CAD build for the part. Positions are in the model's coordinates, mm. Face numbers are marked on the shaded views. A direction names the side the tool comes from. Coordinates: 2 decimals unless noted, no trailing zeros. Write each loop counter-clockwise with the first axis right and the second up, starting at its lowest first coordinate (ties: lowest second). Pieces come first, ordered by that corner, then holes.
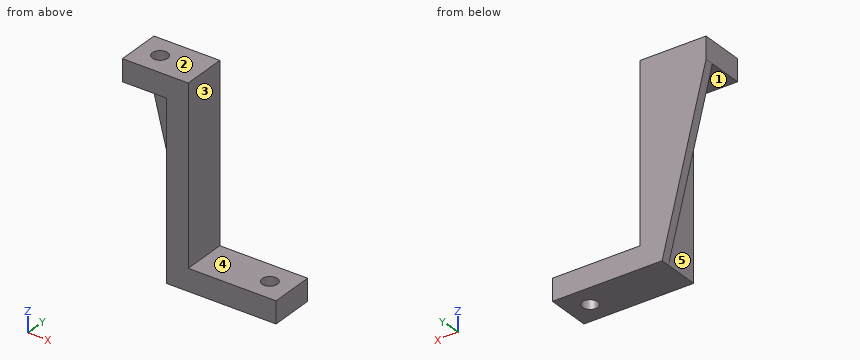
```python
from build123d import *

# Parameters (mm, degrees)
F1_DEPTH = 10
F2_DEPTH = 2
F3_R     = 1.75
F4_DEPTH = 5
F5_R     = 1.75
F6_DEPTH = 5


with BuildPart() as f1:
    # F0 (on Front) → F1 (new body)
    with BuildSketch(Plane.XZ):
        Polygon((0, 40), (-15, 40), (-15, 35), (-5, 35), (-5, -5), (20, -5), (20, 0), (0, 0), align=None)
    extrude(amount=F1_DEPTH)

    # F0 (on Front) → F2 (join)
    with BuildSketch(Plane.XZ):
        Polygon((0, 40), (-15, 40), (-15, 35), (-5, 35), (-5, -5), (20, -5), (20, 0), (0, 0), align=None)
        Polygon((-5, 35), (-15, 35), (-5, -5), align=None)
    extrude(amount=F2_DEPTH)

    # F3 (on face) → F4 (cut)
    with BuildSketch(Plane.XY.offset(40)):
        with Locations((-10, -5)):
            Circle(F3_R)
    extrude(amount=-F4_DEPTH, mode=Mode.SUBTRACT)

    # F5 (on face) → F6 (cut)
    with BuildSketch(Plane.XY):
        with Locations((15, -5)):
            Circle(F5_R)
    extrude(amount=-F6_DEPTH, mode=Mode.SUBTRACT)


solid = f1.part
```
Item 1: Saw through at D-D, the plane x = 15. Write the cut outline in (y, z), and give its area (3 significant figures).
Item 2: Flat gauge pins, fed straight in: pin 1 Ø3 at (x, y) = (15, -5) entering from -Z; pin 2 Ø5 at (y, z) = (-1.5, 3.5) entering from +X; pin 3 Ø4 at (x, y) = (-11, -6.5) entering from -Z; pin 4 Ø2.5 at (y, z) = (-5, 22) entering from -X. Where does each tip first touch, or does it go through?
Item 3: Two-plate mould, pull along X, no slides. Class the marked faces 3, 4 and 5: +X half, -X half, draft (parallel to the pull), parting line (faces both ways), or undercut.
Item 4: Wall check: line 1 along Y through (x, z) = (15, -2); line 2 along X through (y, z) = (-3, 13); line 3 along Z through (x, y) = (-13, -5.5). Give the ranges that are in metal, low to high.
Item 5: Saw through at B-B, the plane x = -10. Write the cut outline in (y, z).
Item 6: Saw through at A-A, the plane y = -5. Write the cut outline in (x, z), and give its area (3 significant figures).
Item 7: Which spindle directions (+Z, -Z, +X, -X, +Y, -Y) get a long thin tool onto all of the face, cutting with end or side? Do the marked faces 1 and 2. Say none if no direction does.
Item 8: Saw through at C-C, the plane z = 29. Write the cut outline in (x, y).
Working result:
1. outline: (-10, -5) - (-6.75, -5) - (-6.75, 0) - (-10, 0) - close; (-3.25, -5) - (0, -5) - (0, 0) - (-3.25, 0) - close
1. area: 32.5 mm2
2. pin 1: passes through
2. pin 2: stops at x = 0
2. pin 3: stops at z = 35
2. pin 4: stops at x = -5
3. face 3: +X half
3. face 4: draft
3. face 5: -X half
4. line 1: y = -10 to -6.75, -3.25 to 0
4. line 2: x = -5 to 0
4. line 3: z = 35 to 40
5. outline: (-10, 35) - (-6.75, 35) - (-6.75, 40) - (-10, 40) - close; (-3.25, 35) - (-2, 35) - (-2, 15) - (0, 15) - (0, 40) - (-3.25, 40) - close
6. outline: (-15, 35) - (-11.75, 35) - (-11.75, 40) - (-15, 40) - close; (-8.25, 35) - (-5, 35) - (-5, -5) - (13.25, -5) - (13.25, 0) - (0, 0) - (0, 40) - (-8.25, 40) - close; (16.75, -5) - (20, -5) - (20, 0) - (16.75, 0) - close
6. area: 340 mm2
7. face 1: -Z, -X, -Y
7. face 2: +Z, +X, -X, +Y, -Y
8. outline: (-13.5, -2) - (-5, -2) - (-5, -10) - (0, -10) - (0, 0) - (-13.5, 0) - close
